The model under review builds one solid part; all positions refer to its coordinate system, in mm. A direction names the side the tool comes from. Round coordinates to 2 decimals unless told otherwise and drop trailing zeros. Order: outer loops, then holes, each group sorted by start corner. A loop starts at its lowest first (then second) coordinate and runs counter-clockwise, first axis right, second up. Notation, with made-up numbers: M 76.5,22.5 L 96.5,22.5 A23 ccw 96.5,30.5 Z; hole C 41.25,34 d2. An arc over 180 degrees is marked long. Answer as a JSON object with one key per item and string values. Group by question number.
1) Consider section A-A, the plane y = 2. Write out the cut boundary in (x, z) (3 decimals).
2) Insertion check: pin 1 Ø4 at (x, z) = (-3.5, 30) entering from -Y; pin 2 Ø3.5 at (x, z) = (-2.5, 10.025) entering from +Y; pin 3 Ø2.5 at (x, z) = (-2.46, -32.83) entering from +Y. Each pin has a flat end and moves straight along its axis. Give the tip position at first contact, or say it passes through.
3) Consider section C-C, the plane y = 4.75. Write out the cut boundary in (x, z) (3 decimals), then the cut area to 3 significant figures.
4) The part is to be moulded in two halves that separate along Z. For faces 1 (the flat face through (1, 4, -28)), 2 (the cylindrical face through (-2.3, 3.13, -11.46)), 3 (the flat face through (-3, 4, 35.131)), 4 (the flat face through (2.587, 4, -34)), say which applies: +Z half, -Z half, draft (parallel to the pull), parting line (faces both ways), or undercut.
5) For faces 5 (the flat face through (2.587, 4, 34)), 6 (the flat face through (2.98, 2.03, -29.66)), 7 (the flat face through (-5, 2, 27)), list the 3-axis set-ups (+Z, -Z, +X, -X, +Y, -Y) from which the entire face can be reached by the end or side of a thin tool; tool diameter is ignored.
6) Consider section B-B, the plane x = 4.5. Write out the cut boundary in (y, z), then the cut area to 3 significant figures.
7) To check wall thickness, follow line 1 (Z direction, x = -4.5, y = 0.5); line 2 (Z direction, x = -2.5, y = 4.5) (3 decimals); line 3 (Z direction, x = 2, y = 0.5). State the ranges of each line that lie inside material, in increasing order.
```python
from build123d import *

# Parameters (mm, degrees)
SKETCH1_W                     = 15
SKETCH1_H                     = 49
BOSS_EXTRUDE1_DEPTH           = 8
CSK_FOR_M3_SFHCS1_D           = 3
CSK_FOR_M3_SFHCS1_CSINK_D     = 6.3
CSK_FOR_M3_SFHCS1_CSINK_ANGLE = 90
BOSS_EXTRUDE2_DEPTH           = 8
BOSS_EXTRUDE3_DEPTH           = 4
BOSS_EXTRUDE4_DEPTH           = 8
SKETCH8_W                     = 10.087191575
SKETCH8_H                     = 5.631262012
BOSS_EXTRUDE5_DEPTH           = 8
CUT_EXTRUDE1_START            = -8
SKETCH9_R                     = 1.5
CUT_EXTRUDE1_DEPTH            = 8


with BuildPart() as part:
    # Sketch1 → Boss-Extrude1 (new body)
    with BuildSketch(Plane(origin=(0, 0, 0), x_dir=(1, 0, 0), z_dir=(0, 1, 0))):
        Rectangle(SKETCH1_W, SKETCH1_H)
    extrude(amount=BOSS_EXTRUDE1_DEPTH)

    # CSK for M3 SFHCS1 (through all)
    with Locations(Plane(origin=(0, 8, 0), x_dir=(1, 0, 0), z_dir=(0, 1, 0))):
        with Locations((-2.499999911, -10.025), (-2.499999911, 9.975)):
            CounterSinkHole(CSK_FOR_M3_SFHCS1_D / 2, CSK_FOR_M3_SFHCS1_CSINK_D / 2, counter_sink_angle=CSK_FOR_M3_SFHCS1_CSINK_ANGLE)

    # Sketch5 → Boss-Extrude2 (add)
    with BuildSketch(Plane(origin=(0, 8, 0), x_dir=(1, 0, 0), z_dir=(0, 1, 0))):
        Polygon((-0.994383151, -24.5), (7.5, -29.368304747), (7.5, -24.5), align=None)
        Polygon((-0.994383151, 24.5), (7.5, 24.5), (7.5, 29.368304747), align=None)
    extrude(amount=-BOSS_EXTRUDE2_DEPTH)

    # Sketch6 → Boss-Extrude3 (add)
    with BuildSketch(Plane(origin=(0, 8, 0), x_dir=(1, 0, 0), z_dir=(0, 1, 0))):
        Polygon((7.5, 29.368304747), (-0.994383151, 24.5), (-7.5, 24.5), (-7.5, 27), (-1.66, 27), (6.256887241, 31.537330028), (7.5, 32.249783379), align=None)
        Polygon((-7.5, -24.5), (-0.994383151, -24.5), (7.5, -29.368304747), (7.5, -32.249783379), (6.256887241, -31.537330028), (-1.66, -27), (-7.5, -27), align=None)
    extrude(amount=-BOSS_EXTRUDE3_DEPTH)

    # Sketch7 → Boss-Extrude4 (add)
    with BuildSketch(Plane(origin=(0, 8, 0), x_dir=(1, 0, 0), z_dir=(0, 1, 0))):
        Polygon((-1.66, -27), (7.5, -32.249783379), (7.5, -35.131262012), (6.256887241, -34.41880866), (-2.325616849, -29.5), (-7.5, -29.5), (-7.5, -27), align=None)
        Polygon((7.5, 32.249783379), (-1.66, 27), (-7.5, 27), (-7.5, 29.5), (-2.325616849, 29.5), (6.256887241, 34.41880866), (7.5, 35.131262012), align=None)
    extrude(amount=-BOSS_EXTRUDE4_DEPTH)

    # Sketch8 → Boss-Extrude5 (add)
    with BuildSketch(Plane(origin=(0, 8, 0), x_dir=(1, 0, 0), z_dir=(0, 1, 0))):
        with Locations((-2.456404213, -32.315631006)):
            Rectangle(SKETCH8_W, SKETCH8_H)
        with Locations((-2.456404213, 32.315631006)):
            Rectangle(SKETCH8_W, SKETCH8_H)
    extrude(amount=-BOSS_EXTRUDE5_DEPTH)

    # Sketch9 → Cut-Extrude1 (cut)
    with BuildSketch(Plane(origin=(0, 8, 0), x_dir=(1, 0, 0), z_dir=(0, 1, 0)).offset(CUT_EXTRUDE1_START)):
        with Locations(Location((-2.456404212, 32.831262012, 0), (0, 0, 270))):
            Circle(SKETCH9_R)
        with Locations(Location((-2.456404212, -32.831262012, 0), (0, 0, 270))):
            Circle(SKETCH9_R)
    extrude(amount=CUT_EXTRUDE1_DEPTH, mode=Mode.SUBTRACT)


solid = part.part
```
Results list:
{
 "1": {"outline": "M -7.5,-35.131 L 2.587,-35.131 L 2.587,-32.316 L 7.5,-35.131 L 7.5,-32.25 L -1.66,-27 L -7.5,-27 Z; M -7.5,-24.5 L -0.994,-24.5 L 7.5,-29.368 L 7.5,29.368 L -0.994,24.5 L -7.5,24.5 Z; M -7.5,27 L -1.66,27 L 7.5,32.25 L 7.5,35.131 L 2.587,32.316 L 2.587,35.131 L -7.5,35.131 Z; hole C -2.5,-9.975 d3; hole C -2.5,10.025 d3; hole C -2.456,-32.831 d3; hole C -2.456,32.831 d3"},
 "2": {"pin 1": "y = 0", "pin 2": "y = 6.6", "pin 3": "through"},
 "3": {"outline": "M -7.5,-35.131 L 2.587,-35.131 L 2.587,-32.316 L 7.5,-35.131 L 7.5,35.131 L 2.587,32.316 L 2.587,35.131 L -7.5,35.131 Z; hole C -2.5,-9.975 d3; hole C -2.5,10.025 d3; hole C -2.456,-32.831 d3; hole C -2.456,32.831 d3", "area": "1,010 mm^2"},
 "4": {"face 1": "undercut", "face 2": "undercut", "face 3": "+Z half", "face 4": "draft"},
 "5": {"face 5": "+Z, +Y, -Y", "face 6": "-Y", "face 7": "-X, -Y"},
 "6": {"outline": "M 0,-33.41 L 8,-33.41 L 8,33.41 L 0,33.41 L 0,30.53 L 4,30.53 L 4,27.65 L 0,27.65 L 0,-27.65 L 4,-27.65 L 4,-30.53 L 0,-30.53 Z", "area": "512 mm^2"},
 "7": {"line 1": "-35.13 to -27, -24.5 to 24.5, 27 to 35.13", "line 2": "-35.131 to -34.331, -31.332 to -11.475, -8.475 to 8.525, 11.525 to 31.332, 34.331 to 35.131", "line 3": "-35.13 to -29.1, -26.22 to 26.22, 29.1 to 35.13"}
}
